```python
from build123d import *
from OCP.BRepFilletAPI import BRepFilletAPI_MakeChamfer

# Parameters (mm, degrees)
SKETCH1_W           = 40.4
SKETCH1_H           = 10
SKETCH1_R           = 2.5
BOSS_EXTRUDE1_DEPTH = 25
SKETCH2_R           = 1.55
CUT_EXTRUDE1_DEPTH  = 34.66065953
CUT_EXTRUDE2_REACH  = 35.661
SKETCH3_R           = 1.25
SKETCH4_R           = 1.25
CUT_EXTRUDE3_DEPTH  = 4
CHAMFER1_SIZE       = 0.891616335
CHAMFER1_SIZE_2     = 1.25
SKETCH5_R           = 3.25
CUT_EXTRUDE4_DEPTH  = 4


with BuildPart() as part:
    # Sketch1 → Boss-Extrude1 (new body)
    with BuildSketch(Plane.XY):
        with Locations((0, 1)):
            Rectangle(SKETCH1_W, SKETCH1_H)
        Circle(SKETCH1_R, mode=Mode.SUBTRACT)
        with Locations((13, 0)):
            Circle(SKETCH1_R, mode=Mode.SUBTRACT)
        with Locations((-13, 0)):
            Circle(SKETCH1_R, mode=Mode.SUBTRACT)
    extrude(amount=BOSS_EXTRUDE1_DEPTH)

    # Sketch2 → Cut-Extrude1 (cut, through all)
    with BuildSketch(Plane(origin=(0, 6, 0), x_dir=(1, 0, 0), z_dir=(0, 1, 0))):
        with Locations(Location((7.5, -18, 0), (0, 0, 180))):
            Circle(SKETCH2_R)
        with Locations(Location((-7.5, -18, 0), (0, 0, 180))):
            Circle(SKETCH2_R)
    extrude(amount=-CUT_EXTRUDE1_DEPTH, mode=Mode.SUBTRACT)

    # Sketch3 → Cut-Extrude2 (cut, up to next)
    with BuildSketch(Plane(origin=(0, 6, 0), x_dir=(1, 0, 0), z_dir=(0, 1, 0)), mode=Mode.PRIVATE) as cut_extrude2_sk1:
        with Locations(Location((0, -3, 0), (0, 0, 180))):
            Circle(SKETCH3_R)
    cut_extrude2_tool1 = extrude(cut_extrude2_sk1.sketch, amount=-CUT_EXTRUDE2_REACH, mode=Mode.PRIVATE) & part.part
    # Sketch3 → Cut-Extrude2 (cut, up to next)
    with BuildSketch(Plane(origin=(0, 6, 0), x_dir=(1, 0, 0), z_dir=(0, 1, 0)), mode=Mode.PRIVATE) as cut_extrude2_sk2:
        with Locations(Location((-12.75, -3, 0), (0, 0, 180))):
            Circle(SKETCH3_R)
    cut_extrude2_tool2 = extrude(cut_extrude2_sk2.sketch, amount=-CUT_EXTRUDE2_REACH, mode=Mode.PRIVATE) & part.part
    # Sketch3 → Cut-Extrude2 (cut, up to next)
    with BuildSketch(Plane(origin=(0, 6, 0), x_dir=(1, 0, 0), z_dir=(0, 1, 0)), mode=Mode.PRIVATE) as cut_extrude2_sk3:
        with Locations(Location((12.75, -3, 0), (0, 0, 180))):
            Circle(SKETCH3_R)
    cut_extrude2_tool3 = extrude(cut_extrude2_sk3.sketch, amount=-CUT_EXTRUDE2_REACH, mode=Mode.PRIVATE) & part.part
    add(cut_extrude2_tool1.solids().sort_by_distance((0, 6, 3))[0], mode=Mode.SUBTRACT)
    add(cut_extrude2_tool2.solids().sort_by_distance((-12.75, 6, 3))[0], mode=Mode.SUBTRACT)
    add(cut_extrude2_tool3.solids().sort_by_distance((12.75, 6, 3))[0], mode=Mode.SUBTRACT)

    # Sketch4 → Cut-Extrude3 (cut)
    with BuildSketch(Plane(origin=(0, 6, 0), x_dir=(1, 0, 0), z_dir=(0, 1, 0))):
        with Locations(Location((-16, -9, 0), (0, 0, 180))):
            Circle(SKETCH4_R)
        with Locations(Location((16, -9, 0), (0, 0, 180))):
            Circle(SKETCH4_R)
    extrude(amount=-CUT_EXTRUDE3_DEPTH, mode=Mode.SUBTRACT)

    # Chamfer1
    chamfer1_edges_1 = [part.edges().sort_by_distance(p)[0] for p in [
        (-14.75, 2, 9),
    ]]
    chamfer1_side_1 = [part.faces().sort_by_distance(p)[0] for p in [
        (-14.75, 2.017832327, 9),
    ]]
    chamfer1_edges_2 = [part.edges().sort_by_distance(p)[0] for p in [
        (17.25, 2, 9),
    ]]
    chamfer1_side_2 = [part.faces().sort_by_distance(p)[0] for p in [
        (17.25, 2.017832327, 9),
    ]]
    chamfer1 = BRepFilletAPI_MakeChamfer(part.part.solid().wrapped)
    for e in chamfer1_edges_1:
        chamfer1.Add(CHAMFER1_SIZE - 0.0001, CHAMFER1_SIZE_2 - 0.0001, e.wrapped, chamfer1_side_1[0].wrapped)
    for e in chamfer1_edges_2:
        chamfer1.Add(CHAMFER1_SIZE - 0.0001, CHAMFER1_SIZE_2 - 0.0001, e.wrapped, chamfer1_side_2[0].wrapped)
    add(Compound.cast(chamfer1.Shape()), mode=Mode.REPLACE)  # a hair under: the kernel refuses the full size

    # Sketch5 → Cut-Extrude4 (cut)
    with BuildSketch(Plane(origin=(0, 6, 0), x_dir=(1, 0, 0), z_dir=(0, 1, 0))):
        with Locations(Location((7.5, -18, 0), (0, 0, 180))):
            Circle(SKETCH5_R)
        with Locations(Location((-7.5, -18, 0), (0, 0, 180))):
            Circle(SKETCH5_R)
    extrude(amount=-CUT_EXTRUDE4_DEPTH, mode=Mode.SUBTRACT)


solid = part.part
```
The model under review builds one solid part; all positions refer to its coordinate system, in mm. A direction names the side the tool comes from. Round coordinates to 2 decimals unless told otherwise and drop trailing zeros. Loops run counter-clockwise (first coordinate to the right, second up) from the corner with the lowest first, then second, coordinate; pieces in that order, holes last. Notation, with made-up numbers: M 36.5,51 L 95.5,51 A18 ccw 95.5,78 Z; hole C 5.25,47.5 d7. An arc over 180 degrees is marked long. Answer as a JSON object with one key per item and string values.
(1) Take a section at D-D on x = 12. Give the boundary of the cut face in (y, z), and give its area (3 significant figures).
Resolved:
{"outline": "M -4,0 L -2.29,0 L -2.29,25 L -4,25 Z; M 2.29,0 L 6,0 L 6,2 L 2.29,2 Z; M 2.29,4 L 6,4 L 6,25 L 2.29,25 Z", "area": "128 mm²"}
(2) Tool access review of faces 4 (the cylindrical face through (11.595, 4.028, 2.521)), 5 (the cylindrical face through (12.46, -2.44, 12.32)): name each direction out of +Z, -Z, +X, -X, +Y, -Y from which nothing blocks a thin tool from reaching the whole face with its end or side.
Resolved:
{"face 4": "+Y", "face 5": "+Z, -Z"}
(3) Take a section at A-A on y = 0. Give the boundary of the cut face in (x, z), and give its area (3 significant figures).
Resolved:
{"outline": "M -20.2,0 L -15.5,0 L -15.5,25 L -20.2,25 Z; M -10.5,0 L -2.5,0 L -2.5,25 L -10.5,25 Z; M 2.5,0 L 10.5,0 L 10.5,25 L 2.5,25 Z; M 15.5,0 L 20.2,0 L 20.2,25 L 15.5,25 Z; hole C -7.5,18 d3.1; hole C 7.5,18 d3.1", "area": "620 mm²"}
(4) To check wall thickness, follow line 1 along X through (y, z) = (3.9, 3); line 2 along Z through (x, y) = (12.75, 4.3); line 3 along X through (y, z) = (-1.25, 8). State the ranges of each line that lie inside material, in increasing order.
Resolved:
{"line 1": "-20.2 to -14, -11.5 to -1.25, 1.25 to 11.5, 14 to 20.2", "line 2": "0 to 1.75, 4.25 to 25", "line 3": "-20.2 to -15.17, -10.83 to -2.17, 2.17 to 10.83, 15.17 to 20.2"}
(5) Clearance check with flat-ended pins moving along their axes: P1, Ø3, axis at x = -12.75, z = 3, coming from the +Y side; P2, Ø2, axis at x = 12.75, z = 3, coming from the +Y side; P3, Ø2, axis at x = -7.5, z = 16.5, coming from the +Y side; P4, Ø1.5, axis at x = 16, z = 9, coming from the +Y side. State where each tip first meets the part, or that it passes through.
Resolved:
{"P1": "y = 6", "P2": "y = -2.17", "P3": "y = 2", "P4": "y = 2.53"}
(6) Take a section at B-B on x = 0. Give the boundary of the cut face in (y, z), and give its area (3 significant figures).
Resolved:
{"outline": "M -4,0 L -2.5,0 L -2.5,25 L -4,25 Z; M 2.5,0 L 6,0 L 6,1.75 L 2.5,1.75 Z; M 2.5,4.25 L 6,4.25 L 6,25 L 2.5,25 Z", "area": "116 mm²"}
(7) Take a section at C-C on x = -7.5. Give the boundary of the cut face in (y, z), and give its area (3 significant figures).
Resolved:
{"outline": "M -4,0 L 6,0 L 6,14.75 L 2,14.75 L 2,16.45 L -4,16.45 Z; M -4,19.55 L 2,19.55 L 2,21.25 L 6,21.25 L 6,25 L -4,25 Z", "area": "205 mm²"}
(8) Draft analysis for pull direction Y (two halves, no side actions). For faces 1 (the conical face through (15.893, 2.142, 9.168)), 2 (the cylindrical face through (-11.5, 4.03, 3.05)), 3 (the cylindrical face through (-13.54, -2.44, 12.32)), state which applies: released by +Y, released by -Y, zero draft, split by the parting line, or undercut.
Resolved:
{"face 1": "released by +Y", "face 2": "zero draft", "face 3": "undercut"}
